```python
from build123d import *

# Parameters (mm, degrees)
F_01_START                                = 3
S01_HEX_COUPLING_BOSS_R                   = 9.8
F_01_HEX_COUPLING_BOSS_DEPTH              = 7.4
F_02_START                                = 6.4
F_02_DRIVE_SPOKE_1_DEPTH                  = 4
S03_FLANGE_STANDOFF_1_R                   = 4.95
F_03_FLANGE_STANDOFF_1_DEPTH              = 6.4
F_04_START                                = 6.4
F_04_DRIVE_SPOKE_2_DEPTH                  = 4
S05_FLANGE_STANDOFF_2_R                   = 4.95
F_05_FLANGE_STANDOFF_2_DEPTH              = 6.4
F_06_START                                = 6.4
F_06_DRIVE_SPOKE_3_DEPTH                  = 4
S07_FLANGE_STANDOFF_3_R                   = 4.95
F_07_FLANGE_STANDOFF_3_DEPTH              = 6.4
F_08_START                                = 0.1
F_08_FLOATING_12_MM_AF_DRIVE_SOCKET_DEPTH = 10.6
F_09_START                                = -0.1
S09_THREE_SHARED_THROUGH_FASTENERS_R      = 1.7
F_09_THREE_SHARED_THROUGH_FASTENERS_DEPTH = 10.6


with BuildPart() as part:
    # S01 - Hex coupling boss → 01 - Hex coupling boss (new body)
    with BuildSketch(Plane.XY.offset(F_01_START)):
        Circle(S01_HEX_COUPLING_BOSS_R)
    extrude(amount=F_01_HEX_COUPLING_BOSS_DEPTH)

    # S02 - Drive spoke 1 → 02 - Drive spoke 1 (add)
    with BuildSketch(Plane.XY.offset(F_02_START)):
        with BuildLine():
            Line((5.901185301, 6.809362547), (27.525849737, 12.603673919))
            ThreePointArc((27.525849737, 12.603673919), (33.710811337, 9.032784674), (30.139922092, 2.847823074))
            Line((30.139922092, 2.847823074), (8.515257656, -2.946488299))
            ThreePointArc((8.515257656, -2.946488299), (2.330296056, 0.624400946), (5.901185301, 6.809362547))
        make_face()
    extrude(amount=F_02_DRIVE_SPOKE_1_DEPTH)

    # S03 - Flange standoff 1 → 03 - Flange standoff 1 (add)
    with BuildSketch(Plane.XY):
        with Locations((28.832885915, 7.725748496)):
            Circle(S03_FLANGE_STANDOFF_1_R)
    extrude(amount=F_03_FLANGE_STANDOFF_1_DEPTH)

    # S04 - Drive spoke 2 → 04 - Drive spoke 2 (add)
    with BuildSketch(Plane.XY.offset(F_04_START)):
        with BuildLine():
            Line((-8.8476736, 1.70589511), (-24.678026663, 17.536248173))
            ThreePointArc((-24.678026663, 17.536248173), (-24.678026663, 24.678026663), (-17.536248173, 24.678026663))
            Line((-17.536248173, 24.678026663), (-1.70589511, 8.8476736))
            ThreePointArc((-1.70589511, 8.8476736), (-1.70589511, 1.70589511), (-8.8476736, 1.70589511))
        make_face()
    extrude(amount=F_04_DRIVE_SPOKE_2_DEPTH)

    # S05 - Flange standoff 2 → 05 - Flange standoff 2 (add)
    with BuildSketch(Plane.XY):
        with Locations((-21.107137418, 21.107137418)):
            Circle(S05_FLANGE_STANDOFF_2_R)
    extrude(amount=F_05_FLANGE_STANDOFF_2_DEPTH)

    # S06 - Drive spoke 3 → 06 - Drive spoke 3 (add)
    with BuildSketch(Plane.XY.offset(F_06_START)):
        with BuildLine():
            Line((2.946488299, -8.515257656), (-2.847823074, -30.139922092))
            ThreePointArc((-2.847823074, -30.139922092), (-9.032784674, -33.710811337), (-12.603673919, -27.525849737))
            Line((-12.603673919, -27.525849737), (-6.809362547, -5.901185301))
            ThreePointArc((-6.809362547, -5.901185301), (-0.624400946, -2.330296056), (2.946488299, -8.515257656))
        make_face()
    extrude(amount=F_06_DRIVE_SPOKE_3_DEPTH)

    # S07 - Flange standoff 3 → 07 - Flange standoff 3 (add)
    with BuildSketch(Plane.XY):
        with Locations((-7.725748496, -28.832885915)):
            Circle(S07_FLANGE_STANDOFF_3_R)
    extrude(amount=F_07_FLANGE_STANDOFF_3_DEPTH)

    # S08 - Floating 12 mm AF drive socket → 08 - Floating 12 mm AF drive socket (cut)
    with BuildSketch(Plane.XY.offset(F_08_START)):
        Polygon((7.216878365, 0), (3.608439182, 6.25), (-3.608439182, 6.25), (-7.216878365, 0), (-3.608439182, -6.25), (3.608439182, -6.25), align=None)
    extrude(amount=F_08_FLOATING_12_MM_AF_DRIVE_SOCKET_DEPTH, mode=Mode.SUBTRACT)

    # S09 - Three shared through-fasteners → 09 - Three shared through-fasteners (cut)
    with BuildSketch(Plane.XY.offset(F_09_START)):
        with Locations((28.832885915, 7.725748496)):
            Circle(S09_THREE_SHARED_THROUGH_FASTENERS_R)
        with Locations((-21.107137418, 21.107137418)):
            Circle(S09_THREE_SHARED_THROUGH_FASTENERS_R)
        with Locations((-7.725748496, -28.832885915)):
            Circle(S09_THREE_SHARED_THROUGH_FASTENERS_R)
    extrude(amount=F_09_THREE_SHARED_THROUGH_FASTENERS_DEPTH, mode=Mode.SUBTRACT)


solid = part.part
```
Input: part model. Units: mm. Frame: model coordinates. A direction names the side the tool comes from. Coordinates: 2 decimals unless noted, no trailing zeros. Write each loop counter-clockwise with the first axis right and the second up, starting at its lowest first coordinate (ties: lowest second). Pieces come first, ordered by that corner, then holes. Notation, with made-up numbers: (19, 89.5) -> (31, 89.5) arc R29 ccw to (31, 127.5) -> close; hole circle Ø5 at (5, 33.5). An arc over 180 degrees is marked (long way). Write each question's results on one line, items separated by ' | '.
Item 1: Section query B-B on y = 11. Return loops of the section in (x, z).
Conclusion:
outline: (-18.14, 6.4) -> (-3.86, 6.4) -> (-3.86, 10.4) -> (-18.14, 10.4) -> close; (21.54, 6.4) -> (25.12, 6.4) -> (25.12, 0) -> (32.55, 0) -> (32.55, 6.4) -> (32.68, 6.4) -> (32.68, 10.4) -> (21.54, 10.4) -> close
Item 2: Section query A-A on z = 1.25. Return loops of the section in (x, y).
Conclusion:
outline: circle Ø9.9 at (-21.11, 21.11); circle Ø9.9 at (-7.73, -28.83); circle Ø9.9 at (28.83, 7.73); hole circle Ø3.4 at (-21.11, 21.11); hole circle Ø3.4 at (-7.73, -28.83); hole circle Ø3.4 at (28.83, 7.73)
Item 3: Pin query (flat end, axial travel): pin 1 Ø6 at (x, y) = (2, -2) entering from -Z; pin 2 Ø6 at (x, z) = (-17, 7.5) entering from -Y; pin 3 Ø2 at (x, z) = (8.5, 4.5) entering from +Y; pin 4 Ø1 at (x, z) = (-19.5, 3.5) entering from -Y. Return the tip coordinate at first contact, or that it passes through.
Conclusion:
pin 1: passes through | pin 2: stops at y = 6.86 | pin 3: stops at y = 6.31 | pin 4: stops at y = 16.28
Item 4: Material intervals for probe 1 along X at (y, z) = (3.5, 6); probe 2 along Y at (x, z) = (-9, 1); probe 3 along Y at (x, z) = (-6.5, 7.5), sorted ascending.
Conclusion:
probe 1: x = -9.15 to -5.2, 5.2 to 9.15, 26.25 to 31.41 | probe 2: y = -33.62 to -29.96, -27.71 to -24.05 | probe 3: y = -33.73 to -30.01, -27.65 to -1.24, 1.24 to 13.64
Item 5: Section query D-D on z = 8.5. Return loops of the section in (x, y), plus the area to 3 significant figures.
Conclusion:
outline: (-24.68, 17.54) -> (-9.51, 2.37) arc R9.8 ccw to (-7.05, -6.81) -> (-12.6, -27.53) arc R5.05 ccw to (-2.85, -30.14) -> (2.7, -9.42) arc R9.8 ccw to (9.42, -2.7) -> (30.14, 2.85) arc R5.05 ccw to (27.53, 12.6) -> (6.81, 7.05) arc R9.8 ccw to (-2.37, 9.51) -> (-17.54, 24.68) arc R5.05 ccw to start; hole circle Ø3.4 at (-21.11, 21.11); hole circle Ø3.4 at (-7.73, -28.83); hole (-7.22, 0) -> (-3.61, -6.25) -> (3.61, -6.25) -> (7.22, 0) -> (3.61, 6.25) -> (-3.61, 6.25) -> close; hole circle Ø3.4 at (28.83, 7.73) | area: 881 mm^2
Item 6: Section query C-C on x = 29. Return loops of the section in (y, z).
Conclusion:
outline: (2.54, 6.4) -> (2.78, 6.4) -> (2.78, 0) -> (6.03, 0) -> (6.03, 10.4) -> (2.54, 10.4) -> close; (9.42, 0) -> (12.67, 0) -> (12.67, 6.4) -> (12.77, 6.4) -> (12.77, 10.4) -> (9.42, 10.4) -> close
Item 7: Set-up query: faces 4 (the flat face through (-5.44, -3.08, 6.65)), 5 (the flat face through (-10.06, 17.2, 8.37)), 6 (the cylindrical face through (-16.386, 22.594, 3.155)), 7 (the flat face through (19.92, 0.11, 8.37)), 8 (the flat face through (-0.1, -6.4, 3)). Return all of +Z, -Z, +X, -X, +Y, -Y with unobstructed straight access to the full face (end or side cutting, diameter ignored); none if empty.
Conclusion:
face 4: +Z, -Z | face 5: +Z, -Z, +Y | face 6: -Z | face 7: +Z, -Z, +X, -Y | face 8: -Z, -X, +Y
Item 8: Mould query, pull axis X, two halves, no side actions, for faces 1 (the cylindrical face through (-8.37, -23.925, 3.155)), 2 (the flat face through (31, 8, 0)), 3 (the flat face through (0, 6.25, 7)). Classes: +X half, -X half, draft (parallel to the pull), parting line (faces both ways), or undercut.
Conclusion:
face 1: parting line | face 2: draft | face 3: undercut
